Can you work these out from the model? Positions are in its coordinate system, mm. Round coordinates to 2 decimals unless told otherwise and drop trailing zeros. Loops run counter-clockwise (first coordinate to the right, second up) from the corner with the lowest first, then second, coordinate; pieces in that order, holes last.
(1) If I drill on line 1 along X through (y, z) = (-31, 6); line 2 along Y through (x, z) = (-50.5, 31.5); line 3 along Y through (x, z) = (-14.5, 12.5), over which ranges is the centre line in solid material (lowest first)?
(2) I want a section at D-D on y = -32. Write out the boundary of the cut face in (x, z), plus the area to 3 significant figures.
(3) I want a section at C-C on z = 18.5. Write out the boundary of the cut face in (x, y).
(4) I want a section at A-A on z = 10. Write out the boundary of the cut face in (x, y), plus the area to 3 significant figures.
(5) Will these pins go through, and if not, where does the flat tip stop? pin 1 Ø5 at (x, z) = (-18, 10.5) entering from -Y; pin 2 Ø5 at (x, z) = (-38, 23.5) entering from -Y; pin 3 Ø10 at (x, z) = (-18.5, 25) entering from +Y.
(6) I want a section at B-B on y = -22. Write out the boundary of the cut face in (x, z), plus the area to 3 significant figures.
from build123d import *

# Parameters (mm, degrees)
F1_DEPTH = 50
F2_R     = 2.5
F3_DEPTH = 93


with BuildPart() as f1:
    # F0 (on Top) → F1 (new body)
    with BuildSketch(Plane.XY):
        Polygon((-4.405333, 7.717764), (-54.404821, 7.944006), (-54.404821, -42.055994), (-51.404821, -42.055994), (-51.404821, 2.944006), (-4.519233, 2.731854), align=None)
    extrude(amount=F1_DEPTH)

    # F2 (on Right) → F3 (cut)
    with BuildSketch(Plane.YZ):
        with Locations((-22.055994, 40)):
            Circle(F2_R)
        with Locations((-22.055994, 10)):
            Circle(F2_R)
    extrude(amount=-F3_DEPTH, mode=Mode.SUBTRACT)


solid = f1.part
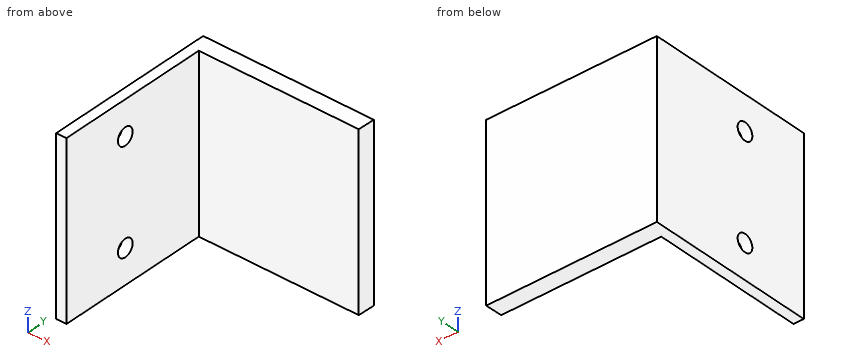
Filled sheet:
1. line 1: x = -54.4 to -51.4
1. line 2: y = 2.94 to 7.93
1. line 3: y = 2.78 to 7.76
2. outline: (-54.4, 0) - (-51.4, 0) - (-51.4, 50) - (-54.4, 50) - close
2. area: 150 mm2
3. outline: (-54.4, -42.06) - (-51.4, -42.06) - (-51.4, 2.94) - (-4.52, 2.73) - (-4.41, 7.72) - (-54.4, 7.94) - close
4. outline: (-54.4, -42.06) - (-51.4, -42.06) - (-51.4, -24.56) - (-54.4, -24.56) - close; (-54.4, -19.56) - (-51.4, -19.56) - (-51.4, 2.94) - (-4.52, 2.73) - (-4.41, 7.72) - (-54.4, 7.94) - close
4. area: 369 mm2
5. pin 1: stops at y = 2.78
5. pin 2: stops at y = 2.87
5. pin 3: stops at y = 7.8
6. outline: (-54.4, 0) - (-51.4, 0) - (-51.4, 7.5) - (-54.4, 7.5) - close; (-54.4, 12.5) - (-51.4, 12.5) - (-51.4, 37.5) - (-54.4, 37.5) - close; (-54.4, 42.5) - (-51.4, 42.5) - (-51.4, 50) - (-54.4, 50) - close
6. area: 120 mm2
